For this review, take the finished solid that the model builds, in its own axes (mm). Face numbers are marked on the shaded views. A direction names the side the tool comes from. Round coordinates to 2 decimals unless told otherwise and drop trailing zeros. Loops run counter-clockwise (first coordinate to the right, second up) from the corner with the lowest first, then second, coordinate; pieces in that order, holes last.
1. Consider section D-D on z = -16.5. State the section outline as (x, y) points.
2. To check wall thickness, follow line 1 along Z through (x, y) = (-54.5, 79); line 2 along Y through (x, z) = (2.5, 3.5); line 3 along Y through (x, z) = (-26, 1.5). State the ranges of each line that lie inside material, in increasing order.
3. Consider section C-C on y = 0. State the section outline as (x, z) points.
4. Tool access review of the marked faces 1 and 2: name each direction out of +Z, -Z, +X, -X, +Y, -Y from which nothing blocks a thin tool from reaching the whole face with its end or side.
5. Consider section B-B on x = 0. State the section outline as (y, z) points, then the cut area to 3 significant figures.
6. Consider section A-A on y = -105.5. State the section outline as (x, z) points, then the cut area to 3 significant figures.
7. Clearance check with flat-ended pins moving along their axes: pin 1 Ø8 at (x, z) = (40, -3.5) entering from +Y; pin 2 Ø1.5 at (x, z) = (-42, 1) entering from +Y; pin 3 Ø3 at (x, y) = (3.5, 10) entering from -Z; pin 4 Ø10 at (x, y) = (52.5, -14.5) entering from -Z. State where each tip first meets the part, or that it passes through.
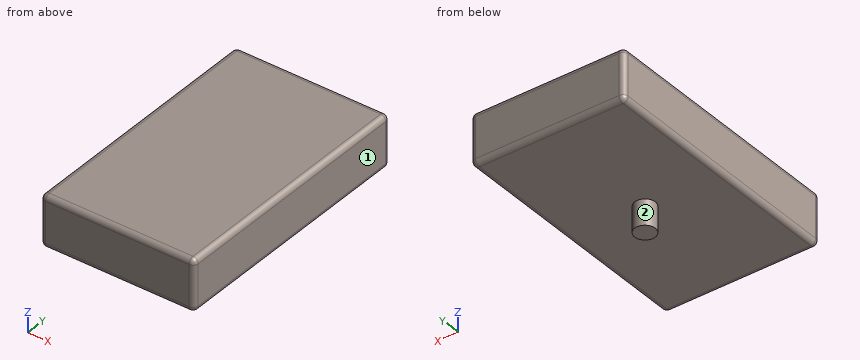
from build123d import *

# Parameters (mm, degrees)
F0_W     = 152.4
F0_H     = 254
F1_DEPTH = 50.8
F2_R     = 5.08
F3_R     = 10.16
F4_DEPTH = 25.4


with BuildPart() as f1:
    # F0 (on Top) → F1 (new body)
    with BuildSketch(Plane.XY):
        Rectangle(F0_W, F0_H)
    extrude(amount=F1_DEPTH)

    # F2
    f2_edges = [f1.edges().sort_by_distance(p)[0] for p in [
        (-76.2, 0, 50.8),
        (-76.2, 127, 25.4),
        (-76.2, 0, 0),
        (-76.2, -127, 25.4),
        (0, -127, 50.8),
        (0, -127, 0),
        (76.2, -127, 25.4),
        (76.2, 0, 50.8),
        (76.2, 0, 0),
        (76.2, 127, 25.4),
        (0, 127, 0),
        (0, 127, 50.8),
    ]]
    fillet(f2_edges, radius=F2_R)

    # F3 (on face) → F4 (join)
    with BuildSketch(Plane(origin=(0, 0, 0), x_dir=(1, 0, 0), z_dir=(0, 0, -1))):
        Circle(F3_R)
    extrude(amount=F4_DEPTH)


solid = f1.part
Resolved:
1. outline: circle Ø20.32 at (0, 0)
2. line 1: z = 0 to 50.8
2. line 2: y = -126.75 to 126.75
2. line 3: y = -125.52 to 125.52
3. outline: (-76.2, 5.08) arc R5.08 ccw to (-71.12, 0) - (-10.16, 0) - (-10.16, -25.4) - (10.16, -25.4) - (10.16, 0) - (71.12, 0) arc R5.08 ccw to (76.2, 5.08) - (76.2, 45.72) arc R5.08 ccw to (71.12, 50.8) - (-71.12, 50.8) arc R5.08 ccw to (-76.2, 45.72) - close
4. face 1: +Z, -Z, +X, +Y, -Y
4. face 2: -Z
5. outline: (-127, 5.08) arc R5.08 ccw to (-121.92, 0) - (-10.16, 0) - (-10.16, -25.4) - (10.16, -25.4) - (10.16, 0) - (121.92, 0) arc R5.08 ccw to (127, 5.08) - (127, 45.72) arc R5.08 ccw to (121.92, 50.8) - (-121.92, 50.8) arc R5.08 ccw to (-127, 45.72) - close
5. area: 13,400 mm2
6. outline: (-76.2, 5.08) arc R5.08 ccw to (-71.12, 0) - (71.12, 0) arc R5.08 ccw to (76.2, 5.08) - (76.2, 45.72) arc R5.08 ccw to (71.12, 50.8) - (-71.12, 50.8) arc R5.08 ccw to (-76.2, 45.72) - close
6. area: 7,720 mm2
7. pin 1: stops at y = 124.12
7. pin 2: stops at y = 125.76
7. pin 3: stops at z = -25.4
7. pin 4: stops at z = 0
